The model under review builds one solid part; all positions refer to its coordinate system, in mm. A direction names the side the tool comes from. Round coordinates to 2 decimals unless told otherwise and drop trailing zeros. Order: outer loops, then holes, each group sorted by start corner. A loop starts at its lowest first (then second) coordinate and runs counter-clockwise, first axis right, second up.
```python
from build123d import *

# Parameters (mm, degrees)
SKETCH1_W            = 100
SKETCH1_H            = 81
SKETCH1_R            = 1.75
SKETCH1_R_2          = 1.575
BOSS_EXTRUDE1_DEPTH  = 3
SKETCH2_W            = 58.5
SKETCH2_H            = 9.2
BOSS_EXTRUDE2_DEPTH  = 18
SKETCH3_W            = 50
SKETCH3_H            = 1.5
BOSS_EXTRUDE3_DEPTH  = 20
SKETCH4_W            = 14.5
SKETCH4_H            = 15
SKETCH4_W_2          = 15
SKETCH4_H_2          = 14.5
BOSS_EXTRUDE4_DEPTH  = 9.25
SKETCH5_W            = 2.5
SKETCH5_H            = 24
BOSS_EXTRUDE5_DEPTH  = 8.5
SKETCH6_W            = 12.1
SKETCH6_H            = 4.1
BOSS_EXTRUDE6_DEPTH  = 2.25
SKETCH6_3_W          = 15.1
SKETCH6_3_H          = 25
BOSS_EXTRUDE7_DEPTH  = 4.25
SKETCH7_R            = 4
BOSS_EXTRUDE8_DEPTH  = 25
SKETCH8_W            = 9.6
SKETCH8_H            = 8.8
BOSS_EXTRUDE9_DEPTH  = 3.95
SKETCH9_W            = 2.2
SKETCH9_H            = 6.72
BOSS_EXTRUDE10_DEPTH = 1.5
SKETCH9_3_W          = 18
SKETCH9_3_H          = 10.7
BOSS_EXTRUDE11_DEPTH = 4.45
SKETCH10_R           = 3.875
BOSS_EXTRUDE12_DEPTH = 22
SKETCH11_W           = 57
SKETCH11_H           = 22.8
BOSS_EXTRUDE13_DEPTH = 21
SKETCH12_W           = 6.8
SKETCH12_H           = 7
BOSS_EXTRUDE14_DEPTH = 8.25
SKETCH13_R           = 0.75
BOSS_EXTRUDE15_DEPTH = 8.7


with BuildPart() as part:
    # Sketch1 → Boss-Extrude1 (new body)
    with BuildSketch(Plane(origin=(0, 0, 0), x_dir=(1, 0, 0), z_dir=(0, 1, 0))):
        Rectangle(SKETCH1_W, SKETCH1_H)
        with Locations(Location((44.8, 36.3, 0), (0, 0, 270))):
            Circle(SKETCH1_R, mode=Mode.SUBTRACT)
        with Locations(Location((3.8, 19.5, 0), (0, 0, 270))):
            Circle(SKETCH1_R, mode=Mode.SUBTRACT)
        with Locations(Location((-44.025, -18.275, 0), (0, 0, 270))):
            Circle(SKETCH1_R_2, mode=Mode.SUBTRACT)
        with Locations(Location((-44.025, -6.875, 0), (0, 0, 270))):
            Circle(SKETCH1_R_2, mode=Mode.SUBTRACT)
    extrude(amount=BOSS_EXTRUDE1_DEPTH)

    # Sketch2 → Boss-Extrude2 (add)
    with BuildSketch(Plane(origin=(0, 3, 0), x_dir=(1, 0, 0), z_dir=(0, 1, 0))):
        with Locations((-17.34, -33.15)):
            Rectangle(SKETCH2_W, SKETCH2_H)
    extrude(amount=BOSS_EXTRUDE2_DEPTH)

    # Sketch3 → Boss-Extrude3 (add)
    with BuildSketch(Plane.XY.offset(37.75)):
        with Locations((-17.34, 16.25)):
            Rectangle(SKETCH3_W, SKETCH3_H)
    extrude(amount=BOSS_EXTRUDE3_DEPTH)

    # Sketch4 → Boss-Extrude4 (add)
    with BuildSketch(Plane(origin=(0, 3, 0), x_dir=(1, 0, 0), z_dir=(0, 1, 0))):
        with Locations((43.75, 22)):
            Rectangle(SKETCH4_W, SKETCH4_H)
        with Locations((4.5, 33.25)):
            Rectangle(SKETCH4_W_2, SKETCH4_H_2)
        with Locations((24.5, 33.25)):
            Rectangle(SKETCH4_W_2, SKETCH4_H_2)
    extrude(amount=BOSS_EXTRUDE4_DEPTH)

    # Sketch5 → Boss-Extrude5 (add)
    with BuildSketch(Plane(origin=(0, 3, 0), x_dir=(1, 0, 0), z_dir=(0, 1, 0))):
        with Locations((-5.65, 26)):
            Rectangle(SKETCH5_W, SKETCH5_H)
    extrude(amount=BOSS_EXTRUDE5_DEPTH)

    # Sketch6 → Boss-Extrude6 (add, symmetric)
    with BuildSketch(Plane(origin=(0, 6.125, 0), x_dir=(1, 0, 0), z_dir=(0, 1, 0))):
        with Locations((4.5, 42.55)):
            Rectangle(SKETCH6_W, SKETCH6_H)
    extrude(amount=BOSS_EXTRUDE6_DEPTH, both=True)

    # Sketch6<3> → Boss-Extrude7 (add, symmetric)
    with BuildSketch(Plane(origin=(0, 6.125, 0), x_dir=(1, 0, 0), z_dir=(0, 1, 0))):
        with Locations((4.5, 57.1)):
            Rectangle(SKETCH6_3_W, SKETCH6_3_H)
    extrude(amount=BOSS_EXTRUDE7_DEPTH, both=True)

    # Sketch7 → Boss-Extrude8 (add)
    with BuildSketch(Plane(origin=(0, 0, -69.6), x_dir=(-1, 0, 0), z_dir=(0, 0, -1))):
        with Locations((-4.5, 6.125)):
            Circle(SKETCH7_R)
    extrude(amount=BOSS_EXTRUDE8_DEPTH)

    # Sketch8 → Boss-Extrude9 (add)
    with BuildSketch(Plane(origin=(0, 3, 0), x_dir=(1, 0, 0), z_dir=(0, 1, 0))):
        with Locations((-43.6, 32.1)):
            Rectangle(SKETCH8_W, SKETCH8_H)
        with Locations((-43.6, 11.7)):
            Rectangle(SKETCH8_W, SKETCH8_H)
    extrude(amount=BOSS_EXTRUDE9_DEPTH)

    # Sketch9 → Boss-Extrude10 (add, symmetric)
    with BuildSketch(Plane(origin=(0, 4.975, 0), x_dir=(1, 0, 0), z_dir=(0, 1, 0))):
        with Locations((-49.5, 11.7)):
            Rectangle(SKETCH9_W, SKETCH9_H)
    extrude(amount=BOSS_EXTRUDE10_DEPTH, both=True)

    # Sketch9<3> → Boss-Extrude11 (add, symmetric)
    with BuildSketch(Plane(origin=(0, 4.975, 0), x_dir=(1, 0, 0), z_dir=(0, 1, 0))):
        with Locations((-59.6, 11.7)):
            Rectangle(SKETCH9_3_W, SKETCH9_3_H)
    extrude(amount=BOSS_EXTRUDE11_DEPTH, both=True)

    # Sketch10 → Boss-Extrude12 (add)
    with BuildSketch(Plane.ZY.offset(68.6)):
        with Locations((-11.7, 4.975)):
            Circle(SKETCH10_R)
    extrude(amount=BOSS_EXTRUDE12_DEPTH)

    # Sketch11 → Boss-Extrude13 (add)
    with BuildSketch(Plane(origin=(0, 3, 0), x_dir=(1, 0, 0), z_dir=(0, 1, 0))):
        with Locations((0, 2.599)):
            Rectangle(SKETCH11_W, SKETCH11_H)
    extrude(amount=BOSS_EXTRUDE13_DEPTH)

    # Sketch12 → Boss-Extrude14 (add)
    with BuildSketch(Plane(origin=(0, 3, 0), x_dir=(1, 0, 0), z_dir=(0, 1, 0))):
        with Locations((42.9, 3.8)):
            Rectangle(SKETCH12_W, SKETCH12_H)
    extrude(amount=BOSS_EXTRUDE14_DEPTH)

    # Sketch13 → Boss-Extrude15 (add)
    with BuildSketch(Plane(origin=(46.3, 0, 0), x_dir=(0, 0, -1), z_dir=(1, 0, 0))):
        with Locations(Location((1.8, 7.125, 0), (0, 0, 180))):
            Circle(SKETCH13_R)
        with Locations(Location((5.8, 7.125, 0), (0, 0, 180))):
            Circle(SKETCH13_R)
    extrude(amount=BOSS_EXTRUDE15_DEPTH)


solid = part.part
```
(1) Consider section B-B (x = -20). Write out the cut boundary in (y, z).
Data:
outline: (0, -40.5) - (3, -40.5) - (3, -14) - (24, -14) - (24, 8.8) - (3, 8.8) - (3, 28.55) - (21, 28.55) - (21, 37.75) - (17, 37.75) - (17, 57.75) - (15.5, 57.75) - (15.5, 37.75) - (3, 37.75) - (3, 40.5) - (0, 40.5) - close
(2) To check wall thickness, follow probe 1 along X at (y, z) = (1.25, -19.5); probe 2 along Z at (x, y) = (-3.5, 5); probe 3 along Y at (x, z) = (24, -23). State the ranges of each line that lie inside material, in increasing order.
Data:
probe 1: x = -50 to 2.05, 5.55 to 50
probe 2: z = -14 to 8.8, 28.55 to 37.75
probe 3: y = 0 to 3
(3) For faces 1 (the flat face through (39.5, 7, -4)), 2 (the flat face through (3, 10, -69.6)), 3 (the flat face through (0, 13, 8.801)), 4 (the flat face through (4, 3.875, -43)), list the 3-axis set-ups (+Z, -Z, +X, -X, +Y, -Y) from which the entire face can be reached by the end or side of a thin tool; tool diameter is ignored.
Data:
face 1: +Z, +Y
face 2: -Z
face 3: +X, -X, +Y
face 4: +X, -X, -Y
(4) Consider section D-D (x = 21). Write out the cut boundary in (y, z), and give its area (3 significant figures).
Data:
outline: (0, -40.5) - (12.25, -40.5) - (12.25, -26) - (3, -26) - (3, -14) - (24, -14) - (24, 8.8) - (3, 8.8) - (3, 40.5) - (0, 40.5) - close
area: 856 mm2
(5) Draft analysis for pull direction X (two halves, no side actions). For faces 5 (the flat face through (11.91, 12, 33)), 6 (the flat face through (-38.8, 5, -32)), 7 (the flat face through (-18, 12, 28.55)), state which applies: pulls with the +X half, pulls with the -X half, needs draft (parallel to the pull), parting line crosses it, or undercut.
Data:
face 5: pulls with the +X half
face 6: undercut
face 7: needs draft
(6) Consider section A-A (z = -19.5). Write out the cut boundary in (x, y), and give its area (3 significant figures).
Data:
outline: (-50, 0) - (2.05, 0) - (2.05, 3) - (-4.4, 3) - (-4.4, 11.5) - (-6.9, 11.5) - (-6.9, 3) - (-50, 3) - close; (5.55, 0) - (50, 0) - (50, 3) - (51, 3) - (51, 12.25) - (36.5, 12.25) - (36.5, 3) - (5.55, 3) - close
area: 445 mm2
(7) Insertion check: pin 1 (4.5 mm diameter, centred on x = -3.5, z = 35, fed in from +Y); pin 2 (8 mm diameter, centred on y = 20.5, z = -18.5, fed in from -X); pin 3 (4.5 mm diameter, centred on x = -44, y = 5, fed in from +Z); pin 4 (1.2 mm diameter, centred on x = -6, y = 6, fed in from -Z). Each pin has a flat end and moves straight along its axis. Give the tip position at first contact, or say it passes through.
Data:
pin 1: stops at y = 21
pin 2: passes through
pin 3: stops at z = 40.5
pin 4: stops at z = -38
